Build history of the part. All positions in model axes, mm. Round coordinates to 2 decimals unless told otherwise and drop trailing zeros. Loops run counter-clockwise (first coordinate to the right, second up) from the corner with the lowest first, then second, coordinate; pieces in that order, holes last.
from build123d import *

# Parameters (mm, degrees)
SKETCH1_R               = 165
BOSS_EXTRUDE1_DEPTH     = 6.35
F_1_4_CLEARANCE_HOLE2_D = 6.7564
SKETCH6_R               = 37.5
CUT_EXTRUDE1_DEPTH      = 7.35


with BuildPart() as part:
    # Sketch1 → Boss-Extrude1 (new body)
    with BuildSketch(Plane(origin=(0, 0, 0), x_dir=(1, 0, 0), z_dir=(0, 1, 0))):
        Circle(SKETCH1_R)
    extrude(amount=BOSS_EXTRUDE1_DEPTH)

    # 1/4 Clearance Hole2 (through all)
    with Locations(Plane(origin=(0, 6.35, 0), x_dir=(1, 0, 0), z_dir=(0, 1, 0))):
        with Locations((-34.85, 34.85), (34.85, -34.85), (34.85, 34.85), (-34.85, -34.85)):
            Hole(F_1_4_CLEARANCE_HOLE2_D / 2)

    # Sketch6 → Cut-Extrude1 (cut, through all)
    with BuildSketch(Plane(origin=(0, 6.35, 0), x_dir=(1, 0, 0), z_dir=(0, 1, 0))):
        Circle(SKETCH6_R)
    extrude(amount=-CUT_EXTRUDE1_DEPTH, mode=Mode.SUBTRACT)


solid = part.part
(1) Slice it at D-D on x = 122. List the corners of the cut face in (y, z).
Responses:
outline: (0, -111.09) - (6.35, -111.09) - (6.35, 111.09) - (0, 111.09) - close
(2) Probe line 1 (Z direction, x = 0, y = 2); line 2 (X direction, y = 1.25, z = 32). List the from-to ranges inside material, lowest first.
Responses:
line 1: z = -165 to -37.5, 37.5 to 165
line 2: x = -161.87 to -36.66, -33.04 to -19.55, 19.55 to 33.04, 36.66 to 161.87
(3) Slice it at B-B on x = 0. List the corners of the cut face in (y, z), plus the area to 3 significant figures.
Responses:
outline: (0, -165) - (6.35, -165) - (6.35, -37.5) - (0, -37.5) - close; (0, 37.5) - (6.35, 37.5) - (6.35, 165) - (0, 165) - close
area: 1,620 mm2
(4) Slice it at A-A on z = 0. List the corners of the cut face in (x, y).
Responses:
outline: (-165, 0) - (-37.5, 0) - (-37.5, 6.35) - (-165, 6.35) - close; (37.5, 0) - (165, 0) - (165, 6.35) - (37.5, 6.35) - close
(5) Slice it at C-C on y = 3.75. List the corners of the cut face in (x, z).
Responses:
outline: circle Ø330 at (0, 0); hole circle Ø6.76 at (-34.85, -34.85); hole circle Ø6.76 at (-34.85, 34.85); hole circle Ø75 at (0, 0); hole circle Ø6.76 at (34.85, -34.85); hole circle Ø6.76 at (34.85, 34.85)
(6) Pin check, flat tips, straight feed: P1, Ø5.5, axis at x = 34.85, z = -34.85, coming from the -Y side; P2, Ø3, axis at x = -18.5, y = 1.5, coming from the -Z side. Stop position of each tip, or through.
Responses:
P1: passes through
P2: stops at z = -164.12
